Geometry: final body of the model. Coordinates: model frame, mm. Give positions to 0.01 mm unless a question says otherwise; leave off trailing zeros. Write each loop counter-clockwise with the first axis right and the second up, starting at its lowest first coordinate (ties: lowest second). Pieces come first, ordered by that corner, then holes. Notation, with made-up numbers: M 70.5,11 L 119.5,11 A5 cw 119.5,18 Z; hole C -25,-29.5 d8. An arc over 180 degrees is marked long. Use one line per item in the form item = value. Start each with the question number.
Item 1: Material intervals for line 1 along X through (y, z) = (0, 6.25); line 2 along X through (y, z) = (16.5, 4.75); line 3 along Y through (x, z) = (8, 0), sorted ascending. Write a range as from..to.
Item 2: Section query B-B on y = 7. Return loops of the section in (x, z) (3 decimals), then the cut area to 3 significant figures.
Item 3: Contact query for flat-ended pins moving along their axis: P1, Ø2, axis at y = 12, z = -1.5, coming from the -X side; P2, Ø2, axis at y = 11.5, z = 0, coming from the -X side; P3, Ø10, axis at x = 12.5, z = -4.5, coming from the +Y side. Output: stop coordinate, or through.
Item 4: Section query A-A on z = -3.75. Return loops of the section in (x, y), then the cut area to 3 significant figures.
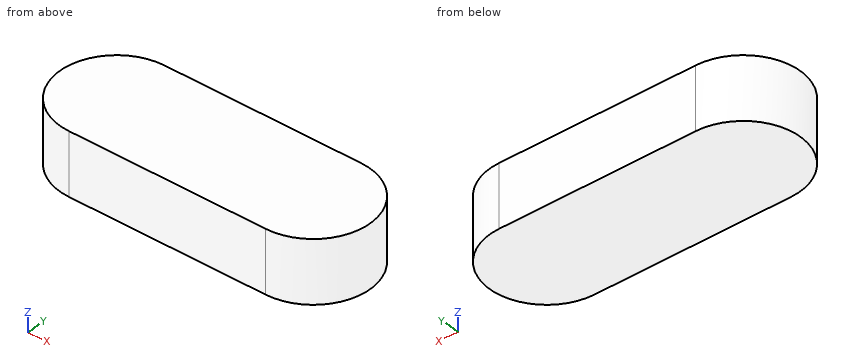
Autodesk Inventor part; units mm, degrees
ref_plane "Work Plane1" through (0, 0, -13) normal (0, 0, 1) x (1, 0, 0)
ref_plane "Work Plane2" through (0, 0, 9) normal (0, 0, 1) x (1, 0, 0)
ref_plane "Work Plane3" through (110, 0, 9) normal (1, 0, 0) x (0, 1, 0)
sketch "Szkic1" plane through (0, 0, 0) normal (0, 0, 1) x (1, 0, 0)
  line L0 (20, 20) -> (90, 20)
  line L1 (90, -20) -> (20, -20)
  arc A0 (20, 20) -> (20, -20) centre (20, 0) ccw
  line L2 (0, 9.4) -> (0, -7.4)
  line L3 (-5, 0) -> (30, 0)
  arc A1 (90, -20) -> (90, 20) centre (90, 0) ccw
  line L4 (110, 0) -> (110, 7) construction
  dimension "d0" = 20
  dimension "d8" = 20
  dimension "d9" = 110
ref_plane "Work Plane1" through (0, 0, -13) normal (0, 0, 1) x (1, 0, 0)
ref_plane "Work Plane2" through (0, 0, 9) normal (0, 0, 1) x (1, 0, 0)
extrude "Bryła1" add sketch "Szkic1" against normal up to surface (22 mm away) from surface at 9
ref_plane "Work Plane3" through (110, 0, 9) normal (1, 0, 0) x (0, 1, 0)
equation "\"d0\" = 0.5 * PB"
equation "\"d8\" = 0.5 * PB"
equation "\"d9\" = NLG"
equation "\"d1\" = -PNT"
equation "\"d2\" = PH - PNT"
equation "\"NLG\" = 110"
equation "\"PNT\" = 13"
equation "\"PH\" = 22"
equation "\"RR\" = 0.001"
equation "\"PHH\" = 0"
equation "\"PUEB\" = 9.4"
properties part number "DIN 6885 - A 40 x 22 x 110" material "Stal, miękka"
Answer sheet:
q1.line_1 = 0..110
q1.line_2 = 8.7..101.3
q1.line_3 = -16..16
q2.outline = M 1.265,-13 L 108.735,-13 L 108.735,9 L 1.265,9 Z
q2.area = 2,360 mm2
q3.P1 = 3.3
q3.P2 = 2.98
q3.P3 = 19.84
q4.outline = M 20,-20 L 90,-20 A20 ccw 90,20 L 20,20 A20 ccw Z
q4.area = 4,060 mm2
